Solid Edge part; units mm, degrees
sketch "Sketch1" plane through (0, 0, 0) normal (1, 0, 0) x (0, 1, 0)
  line L0 (10, -8) -> (45, -8)
  line L1 (45, -8) -> (45, 7)
  line L2 (45, 7) -> (20, 7)
  line L3 (20, 7) -> (10, 15)
  line L4 (10, 15) -> (-7, 7)
  line L5 (0, 0) -> (-7, 7)
  line L6 (0, 0) -> (10, -8)
  dimension "D1" = 45
  dimension "D2" = 45
  dimension "D3" = 10
revolve "RevolvedProtrusion1" add sketch "Sketch1" angle 360 about axis through (0, 56, 17.8505) along (0, 0, -1)
properties material "Steel"
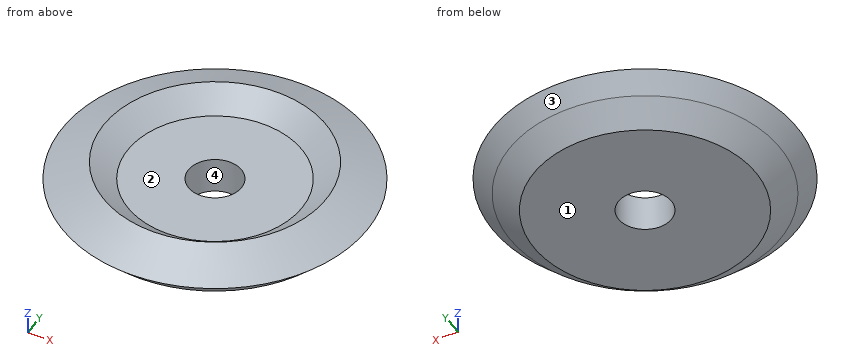
The model under review builds one solid part; all positions refer to its coordinate system, in mm. Face numbers are marked on the shaded views. Round coordinates to 2 decimals unless told otherwise and drop trailing zeros. Loops run counter-clockwise (first coordinate to the right, second up) from the corner with the lowest first, then second, coordinate; pieces in that order, holes last. Notation, with made-up numbers: M 69,29 L 77,29 A24 ccw 77,68 Z; hole C -9,88.25 d5. An arc over 180 degrees is marked long. Answer as a JSON object with one key per item and string values.
Item 1: The part is to be moulded in two halves that separate along Y. For the marked faces 1, 2, 3 and 4, say which applies: +Y half, -Y half, draft (parallel to the pull), parting line (faces both ways), or undercut.
Check sheet entries:
{"face 1": "draft", "face 2": "undercut", "face 3": "parting line", "face 4": "undercut"}
Item 2: Clearance check with flat-ended pins moving along their axes: P1, Ø1, axis at x = -11.5, y = 17, coming from the +Z side; P2, Ø13, axis at x = 0, y = 56, coming from the +Z side; P3, Ø10, axis at y = 45.5, z = 2, coming from the +X side; P4, Ø4, axis at y = 61.5, z = 0.5, coming from the -X side. State where each tip first meets the part, or that it passes through.
Check sheet entries:
{"P1": "z = 11.13", "P2": "through", "P3": "x = 62.18", "P4": "x = -58.25"}
Item 3: We need section C-C, the plane z = 2.5. State the section outline as (x, y) points.
Check sheet entries:
{"outline": "C 0,56 d117; hole C 0,56 d22"}
Item 4: For line 1 along Y through (x, z) = (-15, 7.25); line 2 along Y through (x, z) = (0, -1.5) (3 decimals); line 3 along Z through (x, y) = (-3, 24.5), list the stretches that pass through material, from the lowest coordinate up.
Check sheet entries:
{"line 1": "-4.64 to 22.93, 89.07 to 116.64", "line 2": "1.875 to 45, 67 to 110.125", "line 3": "-8 to 7"}
Item 5: We need section A-A, the plane x = 0. State the section outline as (y, z) points.
Check sheet entries:
{"outline": "M -7,7 L 0,0 L 10,-8 L 45,-8 L 45,7 L 20,7 L 10,15 Z; M 67,-8 L 102,-8 L 112,0 L 119,7 L 102,15 L 92,7 L 67,7 Z"}
Item 6: We need section B-B, the plane y = 56. State the section outline as (x, z) points.
Check sheet entries:
{"outline": "M -63,7 L -56,0 L -46,-8 L -11,-8 L -11,7 L -36,7 L -46,15 Z; M 11,-8 L 46,-8 L 56,0 L 63,7 L 46,15 L 36,7 L 11,7 Z"}
